The model under review builds one solid part; all positions refer to its coordinate system, in mm. Face numbers are marked on the shaded views. A direction names the side the tool comes from. Coordinates: 2 decimals unless noted, no trailing zeros. Write each loop counter-clockwise with the first axis right and the second up, starting at its lowest first coordinate (ties: lowest second). Pieces come first, ordered by that corner, then holes. Notation, with made-up numbers: (74, 17.5) - (114, 17.5) arc R29 ccw to (114, 52.5) - close; hole circle Ø11 at (41, 70). An arc over 180 degrees is marked (long way). Answer as CSV lines item,"result". Start each with the question number.
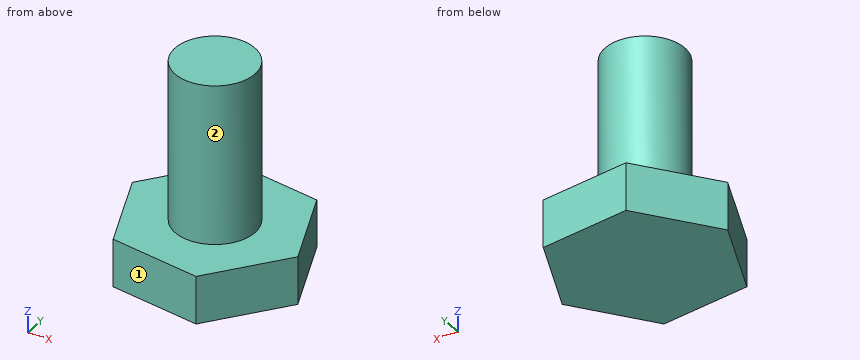
```python
from build123d import *

# Parameters (mm, degrees)
SALIENTE_EXTRUIR3_DEPTH = 3
CROQUIS3_R              = 2.5
SALIENTE_EXTRUIR4_DEPTH = 13


with BuildPart() as part:
    # Croquis1 → Saliente-Extruir3 (new body)
    with BuildSketch(Plane.XY):
        Polygon((-54.386636348, 4.299863782), (-50.772905222, 8.802560828), (-52.865489687, 14.183492308), (-58.571805277, 15.061726742), (-62.185536402, 10.559029696), (-60.092951938, 5.178098216), align=None)
    extrude(amount=SALIENTE_EXTRUIR3_DEPTH)

    # Croquis3 → Saliente-Extruir4 (add)
    with BuildSketch(Plane.XY):
        with Locations((-56.479220812, 9.680795262)):
            Circle(CROQUIS3_R)
    extrude(amount=SALIENTE_EXTRUIR4_DEPTH)


solid = part.part
```
(1) Add section D-D on x = -53.25. Give the boundary of the cut face in (y, z), then the cut area to 3 significant figures.
(2) For the marked faces 1 and 2, list the 3-axis set-ups (+Z, -Z, +X, -X, +Y, -Y) from which the entire face can be reached by the end or side of a thin tool; tool diameter is ignored.
(3) Add section A-A on z = 1. Give the boundary of the cut face in (x, y), then the cut area to 3 significant figures.
(4) Add section C-C on x = -56. Give the boundary of the cut face in (y, z).
(5) For pin 1 (6 mm diameter, centred on y = 11.5, z = 7, fed in from -X); pin 2 (1 mm diameter, centred on y = 11.5, z = 8.5, fed in from -X); pin 3 (3 mm diameter, centred on x = -61, y = 13.5, fed in from -Z); pin 4 (6 mm diameter, centred on y = 13.5, z = 11.5, fed in from -X), all flat-tipped, find the tip position at first contact; note any pin that passes through.
(6) Wall thickness on line 1 (Z direction, x = -55, y = 7); line 2 (X direction, y = 9.75, z = 9.25); line 3 (X direction, y = 10.25, z = 7.25): over which ranges is each line inside the solid? List them lowest first.
(7) Add section B-B on y = 11.75. Give the boundary of the cut face in (x, z), then the cut area to 3 significant figures.
Reported:
1,outline,"(5.72, 0) - (14.24, 0) - (14.24, 3) - (5.72, 3) - close"
1,area,"25.6 mm²"
2,face 1,"+Z, -Z, -X, -Y"
2,face 2,"+Z"
3,outline,"(-62.19, 10.56) - (-60.09, 5.18) - (-54.39, 4.3) - (-50.77, 8.8) - (-52.87, 14.18) - (-58.57, 15.06) - close"
3,area,"86.6 mm²"
4,outline,"(4.55, 0) - (14.67, 0) - (14.67, 3) - (12.13, 3) - (12.13, 13) - (7.23, 13) - (7.23, 3) - (4.55, 3) - close"
5,pin 1,"x = -58.98"
5,pin 2,"x = -58.6"
5,pin 3,"z = 0"
5,pin 4,"x = -58.84"
6,line 1,"0 to 3"
6,line 2,"-58.98 to -53.98"
6,line 3,"-58.91 to -54.04"
7,outline,"(-61.23, 0) - (-51.92, 0) - (-51.92, 3) - (-55.08, 3) - (-55.08, 13) - (-57.88, 13) - (-57.88, 3) - (-61.23, 3) - close"
7,area,"56.0 mm²"
